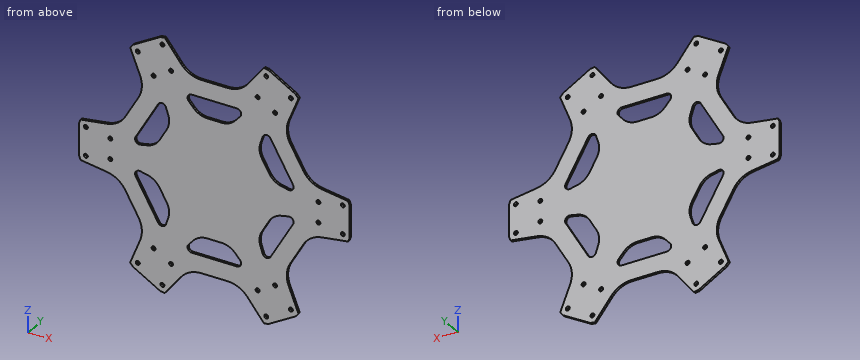
```python
from build123d import *

# Parameters (mm, degrees)
MODEL_R             = 1.625
BOSS_EXTRUDE1_DEPTH = 1.8


with BuildPart() as part:
    # Model → Boss-Extrude1 (new body)
    with BuildSketch(Plane(origin=(0, 0, 0), x_dir=(1, 0, 0), z_dir=(0, 1, 0))):
        with BuildLine():
            Line((-40.455465124, -102.493878505), (-44.082941678, -101.852337067))
            Line((-44.082941678, -101.852337067), (-66.165240495, -89.1031159))
            Line((-66.165240495, -89.1031159), (-68.534569956, -86.282399772))
            Line((-68.534569956, -86.282399772), (-60.482983119, -66.206045102))
            ThreePointArc((-60.482983119, -66.206045102), (-59.040112281, -56.981399894), (-61.775650285, -48.054318215))
            Line((-61.775650285, -48.054318215), (-72.504085478, -29.472123375))
            ThreePointArc((-72.504085478, -29.472123375), (-78.867395992, -22.639537131), (-87.577608502, -19.276777327))
            Line((-87.577608502, -19.276777327), (-108.99003508, -16.211478733))
            Line((-108.99003508, -16.211478733), (-110.248182174, -12.749221166))
            Line((-110.248182174, -12.749221166), (-110.248182174, 12.749221166))
            Line((-110.248182174, 12.749221166), (-108.99003508, 16.211478733))
            Line((-108.99003508, 16.211478733), (-87.577608502, 19.276777327))
            ThreePointArc((-87.577608502, 19.276777327), (-78.867395992, 22.639537131), (-72.504085478, 29.472123375))
            Line((-72.504085478, 29.472123375), (-61.775650285, 48.054318215))
            ThreePointArc((-61.775650285, 48.054318215), (-59.040112281, 56.981399894), (-60.482983119, 66.206045102))
            Line((-60.482983119, 66.206045102), (-68.534569956, 86.282399772))
            Line((-68.534569956, 86.282399772), (-66.165240495, 89.1031159))
            Line((-66.165240495, 89.1031159), (-44.082941678, 101.852337067))
            Line((-44.082941678, 101.852337067), (-40.455465124, 102.493878505))
            Line((-40.455465124, 102.493878505), (-27.094625382, 85.482822428))
            ThreePointArc((-27.094625382, 85.482822428), (-19.82728371, 79.620937024), (-10.728435193, 77.52644159))
            Line((-10.728435193, 77.52644159), (10.728435194, 77.52644159))
            ThreePointArc((10.728435194, 77.52644159), (19.827283711, 79.620937024), (27.094625383, 85.482822428))
            Line((27.094625383, 85.482822428), (40.455465125, 102.493878505))
            Line((40.455465125, 102.493878505), (44.082941679, 101.852337067))
            Line((44.082941679, 101.852337067), (66.165240496, 89.1031159))
            Line((66.165240496, 89.1031159), (68.534569957, 86.282399772))
            Line((68.534569957, 86.282399772), (60.48298312, 66.206045102))
            ThreePointArc((60.48298312, 66.206045102), (59.040112282, 56.981399894), (61.775650286, 48.054318215))
            Line((61.775650286, 48.054318215), (72.504085479, 29.472123375))
            ThreePointArc((72.504085479, 29.472123375), (78.867395993, 22.639537131), (87.577608503, 19.276777327))
            Line((87.577608503, 19.276777327), (108.990035081, 16.211478733))
            Line((108.990035081, 16.211478733), (110.248182175, 12.749221166))
            Line((110.248182175, 12.749221166), (110.248182175, -12.749221166))
            Line((110.248182175, -12.749221166), (108.990035081, -16.211478733))
            Line((108.990035081, -16.211478733), (87.577608503, -19.276777327))
            ThreePointArc((87.577608503, -19.276777327), (78.867395993, -22.639537131), (72.504085479, -29.472123375))
            Line((72.504085479, -29.472123375), (61.775650286, -48.054318215))
            ThreePointArc((61.775650286, -48.054318215), (59.040112282, -56.981399894), (60.48298312, -66.206045102))
            Line((60.48298312, -66.206045102), (68.534569957, -86.282399772))
            Line((68.534569957, -86.282399772), (66.165240496, -89.1031159))
            Line((66.165240496, -89.1031159), (44.082941679, -101.852337067))
            Line((44.082941679, -101.852337067), (40.455465125, -102.493878505))
            Line((40.455465125, -102.493878505), (27.094625383, -85.482822428))
            ThreePointArc((27.094625383, -85.482822428), (19.827283711, -79.620937024), (10.728435194, -77.52644159))
            Line((10.728435194, -77.52644159), (-10.728435193, -77.52644159))
            ThreePointArc((-10.728435193, -77.52644159), (-19.82728371, -79.620937024), (-27.094625382, -85.482822428))
            Line((-27.094625382, -85.482822428), (-40.455465124, -102.493878505))
        make_face()
        with Locations((49.499854453, -69.261690272)):
            Circle(MODEL_R, mode=Mode.SUBTRACT)
        with Locations((35.232456058, -77.498976576)):
            Circle(MODEL_R, mode=Mode.SUBTRACT)
        with Locations((42.287869593, -96.400013533)):
            Circle(MODEL_R, mode=Mode.SUBTRACT)
        with Locations((62.340925848, -84.822376106)):
            Circle(MODEL_R, mode=Mode.SUBTRACT)
        with Locations((84.732310511, 8.237286304)):
            Circle(MODEL_R, mode=Mode.SUBTRACT)
        with Locations((84.732310511, -8.237286304)):
            Circle(MODEL_R, mode=Mode.SUBTRACT)
        with Locations((104.628795441, -11.577637427)):
            Circle(MODEL_R, mode=Mode.SUBTRACT)
        with Locations((104.628795441, 11.577637427)):
            Circle(MODEL_R, mode=Mode.SUBTRACT)
        with Locations((35.232456058, 77.498976576)):
            Circle(MODEL_R, mode=Mode.SUBTRACT)
        with Locations((49.499854453, 69.261690272)):
            Circle(MODEL_R, mode=Mode.SUBTRACT)
        with Locations((62.340925848, 84.822376106)):
            Circle(MODEL_R, mode=Mode.SUBTRACT)
        with Locations((42.287869593, 96.400013533)):
            Circle(MODEL_R, mode=Mode.SUBTRACT)
        with Locations((-49.499854453, 69.261690272)):
            Circle(MODEL_R, mode=Mode.SUBTRACT)
        with Locations((-35.232456058, 77.498976576)):
            Circle(MODEL_R, mode=Mode.SUBTRACT)
        with Locations((-42.287869593, 96.400013533)):
            Circle(MODEL_R, mode=Mode.SUBTRACT)
        with Locations((-62.340925848, 84.822376106)):
            Circle(MODEL_R, mode=Mode.SUBTRACT)
        with Locations((-84.732310511, -8.237286304)):
            Circle(MODEL_R, mode=Mode.SUBTRACT)
        with Locations((-84.732310511, 8.237286304)):
            Circle(MODEL_R, mode=Mode.SUBTRACT)
        with Locations((-104.628795441, 11.577637427)):
            Circle(MODEL_R, mode=Mode.SUBTRACT)
        with Locations((-104.628795441, -11.577637427)):
            Circle(MODEL_R, mode=Mode.SUBTRACT)
        with Locations((-35.232456058, -77.498976576)):
            Circle(MODEL_R, mode=Mode.SUBTRACT)
        with Locations((-49.499854453, -69.261690272)):
            Circle(MODEL_R, mode=Mode.SUBTRACT)
        with Locations((-62.340925848, -84.822376106)):
            Circle(MODEL_R, mode=Mode.SUBTRACT)
        with Locations((-42.287869593, -96.400013533)):
            Circle(MODEL_R, mode=Mode.SUBTRACT)
        with BuildLine():
            Line((18.345415848, -63.41189018), (-18.345415848, -63.41189018))
            ThreePointArc((-18.345415848, -63.41189018), (-21.541027318, -61.339499135), (-20.952320736, -57.576500083))
            Line((-20.952320736, -57.576500083), (-17.005197982, -53.170480885))
            ThreePointArc((-17.005197982, -53.170480885), (-11.951072558, -49.483817856), (-5.832748462, -48.179295586))
            Line((-5.832748462, -48.179295586), (5.832748462, -48.179295586))
            ThreePointArc((5.832748462, -48.179295586), (11.951072558, -49.483817856), (17.005197983, -53.170480885))
            Line((17.005197983, -53.170480885), (20.952320736, -57.576500083))
            ThreePointArc((20.952320736, -57.576500083), (21.541027318, -61.339499135), (18.345415848, -63.41189018))
        make_face(mode=Mode.SUBTRACT)
        with BuildLine():
            Line((64.089015721, -15.818348922), (45.743599874, -47.593541257))
            ThreePointArc((45.743599874, -47.593541257), (42.351050848, -49.324826449), (39.386551365, -46.933492067))
            Line((39.386551365, -46.933492067), (37.544388187, -41.312173892))
            ThreePointArc((37.544388187, -41.312173892), (36.87870706, -35.091841366), (38.808119683, -29.140956135))
            Line((38.808119683, -29.140956135), (44.640868145, -19.038339451))
            ThreePointArc((44.640868145, -19.038339451), (48.829779618, -14.39197649), (54.549586169, -11.858306993))
            Line((54.549586169, -11.858306993), (60.338872101, -10.643008016))
            ThreePointArc((60.338872101, -10.643008016), (63.892078166, -12.014672686), (64.089015721, -15.818348922))
        make_face(mode=Mode.SUBTRACT)
        with BuildLine():
            Line((45.743599874, 47.593541257), (64.089015721, 15.818348922))
            ThreePointArc((64.089015721, 15.818348922), (63.892078166, 12.014672686), (60.338872101, 10.643008016))
            Line((60.338872101, 10.643008016), (54.549586169, 11.858306993))
            ThreePointArc((54.549586169, 11.858306993), (48.829779618, 14.39197649), (44.640868145, 19.038339451))
            Line((44.640868145, 19.038339451), (38.808119683, 29.140956135))
            ThreePointArc((38.808119683, 29.140956135), (36.87870706, 35.091841366), (37.544388187, 41.312173892))
            Line((37.544388187, 41.312173892), (39.386551365, 46.933492067))
            ThreePointArc((39.386551365, 46.933492067), (42.351050848, 49.324826449), (45.743599874, 47.593541257))
        make_face(mode=Mode.SUBTRACT)
        with BuildLine():
            Line((-18.345415848, 63.41189018), (18.345415848, 63.41189018))
            ThreePointArc((18.345415848, 63.41189018), (21.541027318, 61.339499136), (20.952320736, 57.576500083))
            Line((20.952320736, 57.576500083), (17.005197982, 53.170480885))
            ThreePointArc((17.005197982, 53.170480885), (11.951072558, 49.483817856), (5.832748462, 48.179295586))
            Line((5.832748462, 48.179295586), (-5.832748462, 48.179295586))
            ThreePointArc((-5.832748462, 48.179295586), (-11.951072558, 49.483817856), (-17.005197983, 53.170480885))
            Line((-17.005197983, 53.170480885), (-20.952320736, 57.576500083))
            ThreePointArc((-20.952320736, 57.576500083), (-21.541027318, 61.339499136), (-18.345415848, 63.41189018))
        make_face(mode=Mode.SUBTRACT)
        with BuildLine():
            Line((-64.089015722, 15.818348923), (-45.743599874, 47.593541257))
            ThreePointArc((-45.743599874, 47.593541257), (-42.351050848, 49.324826449), (-39.386551365, 46.933492067))
            Line((-39.386551365, 46.933492067), (-37.544388187, 41.312173892))
            ThreePointArc((-37.544388187, 41.312173892), (-36.87870706, 35.091841366), (-38.808119683, 29.140956135))
            Line((-38.808119683, 29.140956135), (-44.640868145, 19.038339451))
            ThreePointArc((-44.640868145, 19.038339451), (-48.829779618, 14.39197649), (-54.549586169, 11.858306993))
            Line((-54.549586169, 11.858306993), (-60.338872101, 10.643008016))
            ThreePointArc((-60.338872101, 10.643008016), (-63.892078166, 12.014672686), (-64.089015722, 15.818348923))
        make_face(mode=Mode.SUBTRACT)
        with BuildLine():
            Line((-45.743599874, -47.593541257), (-64.089015722, -15.818348923))
            ThreePointArc((-64.089015722, -15.818348923), (-63.892078166, -12.014672686), (-60.338872101, -10.643008016))
            Line((-60.338872101, -10.643008016), (-54.549586169, -11.858306993))
            ThreePointArc((-54.549586169, -11.858306993), (-48.829779618, -14.39197649), (-44.640868145, -19.038339451))
            Line((-44.640868145, -19.038339451), (-38.808119683, -29.140956135))
            ThreePointArc((-38.808119683, -29.140956135), (-36.87870706, -35.091841366), (-37.544388187, -41.312173892))
            Line((-37.544388187, -41.312173892), (-39.386551365, -46.933492067))
            ThreePointArc((-39.386551365, -46.933492067), (-42.351050848, -49.324826449), (-45.743599874, -47.593541257))
        make_face(mode=Mode.SUBTRACT)
    extrude(amount=BOSS_EXTRUDE1_DEPTH)


solid = part.part
```
Input: part model. Units: mm. Frame: model coordinates. Give positions to 0.01 mm unless a question says otherwise; leave off trailing zeros. Order: outer loops, then holes, each group sorted by start corner. A loop starts at its lowest first (then second) coordinate and runs counter-clockwise, first axis right, second up. Notation, with made-up numbers: (83.25, -20.75) -> (115.25, -20.75) arc R31 cw to (115.25, 15.25) -> close; hole circle Ø1 at (1.25, 51). An arc over 180 degrees is marked (long way). Write each question's results on one line, items separated by ' | '. Start each with the question number.
Item 1: Cut plane C-C on y = 1.3. Give the number of separate pieces and of enclosed holes in the cut face, then the cut area to 3 significant figures.
Item 2: Contact query for flat-ended pins moving along their axis: P1, Ø0.9, axis at x = 8.5, y = 1, coming from the -Z side; P2, Ø2.5, axis at x = 104.63, z = -11.58, coming from the +Y side; P3, Ø1, axis at y = 1, z = 45, coming from the +X side. Output: stop coordinate, or through.
Item 3: Cut plane B-B on z = -32. Return the cut outline in (x, y), then the cut area to 3 significant figures.
Item 4: Cut plane D-D on x = 92. Return the cut outline in (y, z), then the cut area to 3 significant figures.
Item 5: Cut plane A-A on x = -1. Return the cut outline in (y, z), then the cut area to 3 significant figures.
Item 6: Line query: line 1 (Z direction, x = -1, y = 0.45); line 2 (Z direction, x = 55.5, y = 1.2); line 3 (X direction, y = 1.75, z = -35.5). Output: solid intervals per line, ascending.
Established:
1) separate pieces: 1 | enclosed holes: 30 | area: 23,200 mm^2
2) P1: z = -77.53 | P2: through | P3: x = 63.83
3) outline: (-71.04, 0) -> (-54.75, 0) -> (-54.75, 1.8) -> (-71.04, 1.8) -> close; (-37.53, 0) -> (37.53, 0) -> (37.53, 1.8) -> (-37.53, 1.8) -> close; (54.75, 0) -> (71.04, 0) -> (71.04, 1.8) -> (54.75, 1.8) -> close | area: 194 mm^2
4) outline: (0, -18.64) -> (1.8, -18.64) -> (1.8, 18.64) -> (0, 18.64) -> close | area: 67.1 mm^2
5) outline: (0, -77.53) -> (1.8, -77.53) -> (1.8, -63.41) -> (0, -63.41) -> close; (0, -48.18) -> (1.8, -48.18) -> (1.8, 48.18) -> (0, 48.18) -> close; (0, 63.41) -> (1.8, 63.41) -> (1.8, 77.53) -> (0, 77.53) -> close | area: 224 mm^2
6) line 1: -77.53 to -63.41, -48.18 to 48.18, 63.41 to 77.53 | line 2: -95.26 to -30.69, -11.66 to 11.66, 30.69 to 95.26 | line 3: -69.02 to -52.73, -36.84 to 36.84, 52.73 to 69.02
